```python
from build123d import *

# Parameters (mm, degrees)
ESQUISSE1_R             = 2.5
BOSS_EXTRU_1_DEPTH      = 80
ESQUISSE2_R             = 3.5
BOSS_EXTRU_2_DEPTH      = 3
ESQUISSE3_W             = 30
ESQUISSE3_H             = 5
ENL_V_MAT_EXTRU_1_DEPTH = 3
ESQUISSE4_R             = 1
ENL_V_MAT_EXTRU_2_DEPTH = 1.5


with BuildPart() as part:
    # Esquisse1 → Boss.-Extru.1 (new body)
    with BuildSketch(Plane.XY):
        Circle(ESQUISSE1_R)
    extrude(amount=BOSS_EXTRU_1_DEPTH)

    # Esquisse2 → Boss.-Extru.2 (add)
    with BuildSketch(Plane(origin=(0, 0, 0), x_dir=(-1, 0, 0), z_dir=(0, 0, -1))):
        Circle(ESQUISSE2_R)
    extrude(amount=BOSS_EXTRU_2_DEPTH)

    # Esquisse3 → Enlèv. mat.-Extru.1 (cut)
    with BuildSketch(Plane(origin=(1, 0, 0), x_dir=(0, 0, -1), z_dir=(1, 0, 0))):
        with Locations((-25, 0)):
            Rectangle(ESQUISSE3_W, ESQUISSE3_H)
    extrude(amount=ENL_V_MAT_EXTRU_1_DEPTH, mode=Mode.SUBTRACT)

    # Esquisse4 → Enlèv. mat.-Extru.2 (cut)
    with BuildSketch(Plane(origin=(1, 0, 0), x_dir=(0, 0, -1), z_dir=(1, 0, 0))):
        with Locations((-30, 0)):
            Circle(ESQUISSE4_R)
        with Locations((-20, 0)):
            Circle(ESQUISSE4_R)
    extrude(amount=-ENL_V_MAT_EXTRU_2_DEPTH, mode=Mode.SUBTRACT)


solid = part.part
```
Input: part model. Units: mm. Frame: model coordinates. A direction names the side the tool comes from. Give positions to 0.01 mm unless a question says otherwise; leave off trailing zeros. Order: outer loops, then holes, each group sorted by start corner. A loop starts at its lowest first (then second) coordinate and runs counter-clockwise, first axis right, second up. Notation, with made-up numbers: (-9, 81) - (46, 81) arc R27 ccw to (46, 108) - close; hole circle Ø6 at (-32, 38.5). An arc over 180 degrees is marked (long way). One line per item, written item: value.
1. Cut plane C-C, the plane x = 0.25. Output: boundary loops of the cut face in (y, z).
Determined:
outline: (-3.49, -3) - (3.49, -3) - (3.49, 0) - (2.49, 0) - (2.49, 80) - (-2.49, 80) - (-2.49, 0) - (-3.49, 0) - close; hole circle Ø2 at (0, 20); hole circle Ø2 at (0, 30)
2. Draft query along Z for faces 6 (the face through (0, 0, -3)), 7 (the face through (0, 0, 21)), 8 (the face through (-2, -2, 0)), 9 (the face through (-0.5, 0, 20)). Return one class per face: released by +Z, released by -Z, zero draft, split by the parting line, or undercut.
Determined:
face 6: released by -Z
face 7: undercut
face 8: released by +Z
face 9: undercut
3. Cut plane B-B, the plane z = 20. Output: boundary loops of the cut face in (x, y), and give its area (3 significant figures).
Determined:
outline: (-0.5, -1) - (-0.5, 1) - (1, 1) - (1, 2.29) arc R2.5 ccw (long way) to (1, -2.29) - (1, -1) - close
area: 11.7 mm2
4. Line query: probe 1 along Y at (x, z) = (-0.2, 20); probe 2 along X at (y, z) = (1, 16); probe 3 along X at (y, z) = (-1, 2.5). Output: solid intervals per line, ascending.
Determined:
probe 1: -2.49 to -1, 1 to 2.49
probe 2: -2.29 to 1
probe 3: -2.29 to 2.29
5. Reachability of faces 1 (the face through (-2.5, 0.1, 39.4)), 2 (the face through (0, 0, 29)), 3 (the face through (-3.233, -1.341, -1.479)), 4 (the face through (0, 0, 80)), 5 (the face through (2, 0, 40)) from +Z, -Z, +X, -X, +Y, -Y: full face, straight path, thin tool, end or side. Return the list, or none.
Determined:
face 1: +Z
face 2: +X
face 3: +Z, -Z
face 4: +Z, +X, -X, +Y, -Y
face 5: +X, +Y, -Y
6. Pin query (flat end, axial travel): pin 1 Ø1.4 at (y, z) = (0.5, 17.5) entering from +X; pin 2 Ø1.8 at (y, z) = (0, 30) entering from -X; pin 3 Ø0.6 at (y, z) = (0, 30.5) entering from +X. Return the tip coordinate at first contact, or that it passes through.
Determined:
pin 1: x = 1
pin 2: x = -2.5
pin 3: x = -0.5
7. Cut plane D-D, the plane z = 65.5. Output: boundary loops of the cut face in (x, y), and give its area (3 significant figures).
Determined:
outline: circle Ø5 at (0, 0)
area: 19.6 mm2
8. Cut plane A-A, the plane y = 0. Output: boundary loops of the cut face in (x, z), and give its area (3 significant figures).
Determined:
outline: (-3.5, -3) - (3.5, -3) - (3.5, 0) - (2.5, 0) - (2.5, 10) - (1, 10) - (1, 19) - (-0.5, 19) - (-0.5, 21) - (1, 21) - (1, 29) - (-0.5, 29) - (-0.5, 31) - (1, 31) - (1, 40) - (2.5, 40) - (2.5, 80) - (-2.5, 80) - (-2.5, 0) - (-3.5, 0) - close
area: 370 mm2
